The model under review builds one solid part; all positions refer to its coordinate system, in mm. A direction names the side the tool comes from. Give positions to 0.01 mm unless a question says otherwise; leave off trailing zeros. Write each loop counter-clockwise with the first axis right and the second up, starting at its lowest first coordinate (ties: lowest second). Pieces come first, ordered by that corner, then holes.
from build123d import *

# Parameters (mm, degrees)
CHAMFER_2_SIZE      = 3
SKETCH_4_R          = 3.5
CUT_EXTRUDE_1_DEPTH = 10
SKETCH_5_R          = 82
SKETCH_5_R_2        = 81
EXTRUDE_1_DEPTH     = 1


with BuildPart() as part:
    # 草图2 → 旋转1 (revolve)
    with BuildSketch(Plane.XY, mode=Mode.PRIVATE) as revolve_1_sk:
        Polygon((10, 81), (150, 81), (150, 86), (150, 96), (120, 96), (75, 86), (10, 86), align=None)
    revolve(revolve_1_sk.sketch.rotate(Axis((0, 0, 0), (1, 0, 0)), 90), axis=Axis((0, 0, 0), (1, 0, 0)))

    # 倒角2
    chamfer_2_edges = [part.edges().sort_by_distance(p)[0] for p in [
        (10, 0, -86),
    ]]
    chamfer(chamfer_2_edges, length=CHAMFER_2_SIZE)

    # 草图4 → 切除-拉伸1 (cut)
    with BuildSketch(Plane(origin=(150, 0, 0), x_dir=(0, 0, -1), z_dir=(1, 0, 0))):
        with Locations((44.25, 76.643248235)):
            Circle(SKETCH_4_R)
        with Locations((0, 88.5)):
            Circle(SKETCH_4_R)
        with Locations((76.643248235, 44.25)):
            Circle(SKETCH_4_R)
        with Locations((88.5, 0)):
            Circle(SKETCH_4_R)
        with Locations((76.643248235, -44.25)):
            Circle(SKETCH_4_R)
        with Locations((44.25, -76.643248235)):
            Circle(SKETCH_4_R)
        with Locations((0, -88.5)):
            Circle(SKETCH_4_R)
        with Locations((-44.25, -76.643248235)):
            Circle(SKETCH_4_R)
        with Locations((-76.643248235, -44.25)):
            Circle(SKETCH_4_R)
        with Locations((-88.5, 0)):
            Circle(SKETCH_4_R)
        with Locations((-76.643248235, 44.25)):
            Circle(SKETCH_4_R)
        with Locations((-44.25, 76.643248235)):
            Circle(SKETCH_4_R)
    extrude(amount=-CUT_EXTRUDE_1_DEPTH, mode=Mode.SUBTRACT)

    # 草图5 → 凸台-拉伸1 (add)
    with BuildSketch(Plane(origin=(150, 0, 0), x_dir=(0, 0, -1), z_dir=(1, 0, 0))):
        with Locations(Location((0, 0, 0), (0, 0, 180))):
            Circle(SKETCH_5_R)
        with Locations(Location((0, 0, 0), (0, 0, 180))):
            Circle(SKETCH_5_R_2, mode=Mode.SUBTRACT)
    extrude(amount=EXTRUDE_1_DEPTH)


solid = part.part
1) Consider section C-C, the plane x = 48. Give the boundary of the cut face in (y, z).
2) Tool access review of faces 4 (the cylindrical face through (145.07, -43.199, 73.305)), 5 (the cylindrical face through (43.566, -85.268, -11.195)): name each direction out of +Z, -Z, +X, -X, +Y, -Y from which nothing blocks a thin tool from reaching the whole face with its end or side.
3) Consider section A-A, the plane y = 0. Give the boundary of the cut face in (x, z), then the cut area to 3 significant figures.
4) To check wall thickness, follow probe 1 along Y at (x, z) = (144.75, 0); probe 2 along Y at (x, z) = (63, 0); probe 3 along Y at (x, z) = (145, -44). State the ranges of each line that lie inside material, in increasing order.
5) Consider section D-D, the plane x = 99. Give the boundary of the cut face in (y, z), then the cut area to 3 significant figures.
6) Insertion check: pin 1 (9 mm diameter, centred on y = -76.64, z = 44.25, fed in from -X); pin 2 (7.5 mm diameter, centred on y = -77, z = 45, fed in from +X); pin 3 (10 mm diameter, centred on y = -13, z = 71.5, fed in from -X); pin 4 (3.5 mm diameter, centred on y = 87, z = 0, fed in from +X). Each pin has a flat end and moves straight along its axis. Give the tip position at first contact, or say it passes through.
7) The part is to be moulded in two halves that separate along Y. For faces 1 (the flat face through (140, 44, 77)), 2 (the cylindrical face through (150.493, 31.406, 75.747)), 3 (the flat face through (150, 71, -42)), say which applies: +Y half, -Y half, draft (parallel to the pull), parting line (faces both ways), or undercut.
Answer block:
1. outline: circle Ø172 at (0, 0); hole circle Ø162 at (0, 0)
2. face 4: +X
2. face 5: -X
3. outline: (10, -83) - (13, -86) - (75, -86) - (120, -96) - (150, -96) - (150, -92) - (140, -92) - (140, -85) - (150, -85) - (150, -82) - (151, -82) - (151, -81) - (10, -81) - close; (10, 81) - (151, 81) - (151, 82) - (150, 82) - (150, 85) - (140, 85) - (140, 92) - (150, 92) - (150, 96) - (120, 96) - (75, 86) - (13, 86) - (10, 83) - close
3. area: 2,300 mm2
4. probe 1: y = -96 to -92, -85 to -81, 81 to 85, 92 to 96
4. probe 2: y = -86 to -81, 81 to 86
4. probe 3: y = -85.32 to -80.13, -73.15 to -68.01, 68.01 to 73.15, 80.13 to 85.32
5. outline: circle Ø182.67 at (0, 0); hole circle Ø162 at (0, 0)
5. area: 5,590 mm2
6. pin 1: stops at x = 11
6. pin 2: stops at x = 150
6. pin 3: passes through
6. pin 4: stops at x = 140
7. face 1: undercut
7. face 2: parting line
7. face 3: draft
